from build123d import *

# Parameters (mm, degrees)
PAD019_DEPTH = 40
SKETCH075_W  = 320
SKETCH075_H  = 40
PAD020_DEPTH = 40
SKETCH076_W  = 320
SKETCH076_H  = 40
PAD021_DEPTH = 40
PAD022_DEPTH = 40
SKETCH078_W  = 1120
SKETCH078_H  = 40
PAD023_DEPTH = 40


with BuildPart() as part:
    # Sketch074 (on Face1 of Binder024) → Pad019 (new body)
    with BuildSketch(Plane.XZ.offset(2.1)):
        Polygon((-300, -343.2), (900, -343.2), (900, -943.2), (860, -943.2), (860, -383.2), (-260, -383.2), (-260, -943.2), (-300, -943.2), align=None)
    extrude(amount=-PAD019_DEPTH)

    # Sketch075 (on Face2 of Pad019) → Pad020 (join)
    with BuildSketch(Plane.YZ.offset(900)):
        with Locations((197.9, -363.2)):
            Rectangle(SKETCH075_W, SKETCH075_H)
        with Locations((197.9, -923.2)):
            Rectangle(SKETCH075_W, SKETCH075_H)
    extrude(amount=-PAD020_DEPTH)

    # Sketch076 (on Face1 of Pad020) → Pad021 (join)
    with BuildSketch(Plane(origin=(-300, 0, 0), x_dir=(0, -1, 0), z_dir=(-1, 0, 0))):
        with Locations((-197.9, -363.2)):
            Rectangle(SKETCH076_W, SKETCH076_H)
        with Locations((-197.9, -923.2)):
            Rectangle(SKETCH076_W, SKETCH076_H)
    extrude(amount=-PAD021_DEPTH)

    # Sketch077 (on Face9 of Pad021) → Pad022 (join)
    with BuildSketch(Plane(origin=(0, 357.9, 0), x_dir=(-1, 0, 0), z_dir=(0, 1, 0))):
        Polygon((-900, -943.2), (-900, -343.2), (300, -343.2), (300, -943.2), (260, -943.2), (260, -383.2), (-860, -383.2), (-860, -943.2), align=None)
    extrude(amount=-PAD022_DEPTH)

    # Sketch078 (on Face2 of Pad022) → Pad023 (join)
    with BuildSketch(Plane(origin=(0, 0, -383.2), x_dir=(1, 0, 0), z_dir=(0, 0, -1))):
        with Locations((300, -177.9)):
            Rectangle(SKETCH078_W, SKETCH078_H)
    extrude(amount=-PAD023_DEPTH)


solid = part.part
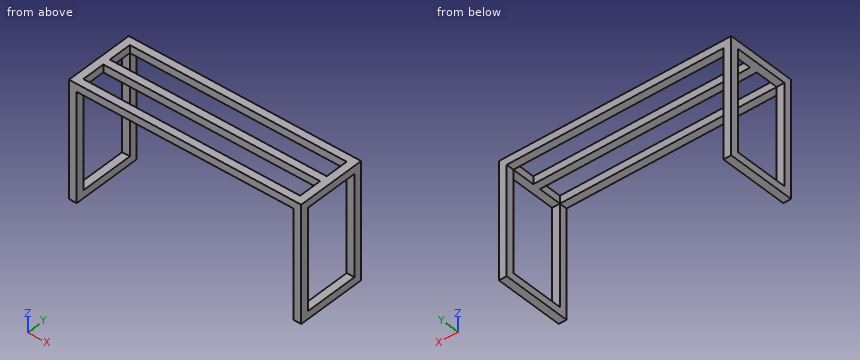
Verification items for the finished model (mm, model axes). Round coordinates to 2 decimals unless told otherwise and drop trailing zeros. Loops run counter-clockwise (first coordinate to the right, second up) from the corner with the lowest first, then second, coordinate; pieces in that order, holes last. Notation, with made-up numbers: (20.25, -39) - (68.25, -39) arc R11 cw to (68.25, -21) - close; hole circle Ø5 at (28.5, 52.25). An arc over 180 degrees is marked (long way). Use a Markdown table: item, result. Add a question column.
1. Section check B-B, the plane y = 142.5. Record the boundary of the cut face in (x, z), plus the area to 3 significant figures.
2. Gauge pin test, flat end, axial feed: pin 1 (12 mm diameter, centred on x = 100.5, y = 338, fed in from -Z). Record the tip position at first contact, or that the pin passes through.
3. Section check C-C, the plane z = -478. Record the boundary of the cut face in (x, y), plus the area to 3 significant figures.
4. Thickness scan on probe 1 along Y at (x, z) = (92, -381); probe 2 along X at (y, z) = (63, -916); probe 3 along Z at (x, y) = (-3.5, 341.5). Record the ranges inside material, lowest first. Write a range as [from, to].
5. Section check D-D, the plane y = 333. Record the boundary of the cut face in (x, z).
6. Section check A-A, the plane x = -24. Record the boundary of the cut face in (y, z), plus the area to 3 significant figures.
Checks:
| question | item | result |
|---|---|---|
| 1 | outline | (-300, -943.2) - (-260, -943.2) - (-260, -903.2) - (-300, -903.2) - close; (-300, -383.2) - (-260, -383.2) - (-260, -343.2) - (-300, -343.2) - close; (860, -943.2) - (900, -943.2) - (900, -903.2) - (860, -903.2) - close; (860, -383.2) - (900, -383.2) - (900, -343.2) - (860, -343.2) - close |
| 1 | area | 6,400 mm^2 |
| 2 | pin 1 | stops at z = -383.2 |
| 3 | outline | (-300, -2.1) - (-260, -2.1) - (-260, 37.9) - (-300, 37.9) - close; (-300, 317.9) - (-260, 317.9) - (-260, 357.9) - (-300, 357.9) - close; (860, -2.1) - (900, -2.1) - (900, 37.9) - (860, 37.9) - close; (860, 317.9) - (900, 317.9) - (900, 357.9) - (860, 357.9) - close |
| 3 | area | 6,400 mm^2 |
| 4 | probe 1 | y = [-2.1, 37.9], [157.9, 197.9], [317.9, 357.9] |
| 4 | probe 2 | x = [-300, -260], [860, 900] |
| 4 | probe 3 | z = [-383.2, -343.2] |
| 5 | outline | (-300, -943.2) - (-260, -943.2) - (-260, -383.2) - (860, -383.2) - (860, -943.2) - (900, -943.2) - (900, -343.2) - (-300, -343.2) - close |
| 6 | outline | (-2.1, -383.2) - (37.9, -383.2) - (37.9, -343.2) - (-2.1, -343.2) - close; (157.9, -383.2) - (197.9, -383.2) - (197.9, -343.2) - (157.9, -343.2) - close; (317.9, -383.2) - (357.9, -383.2) - (357.9, -343.2) - (317.9, -343.2) - close |
| 6 | area | 4,800 mm^2 |
